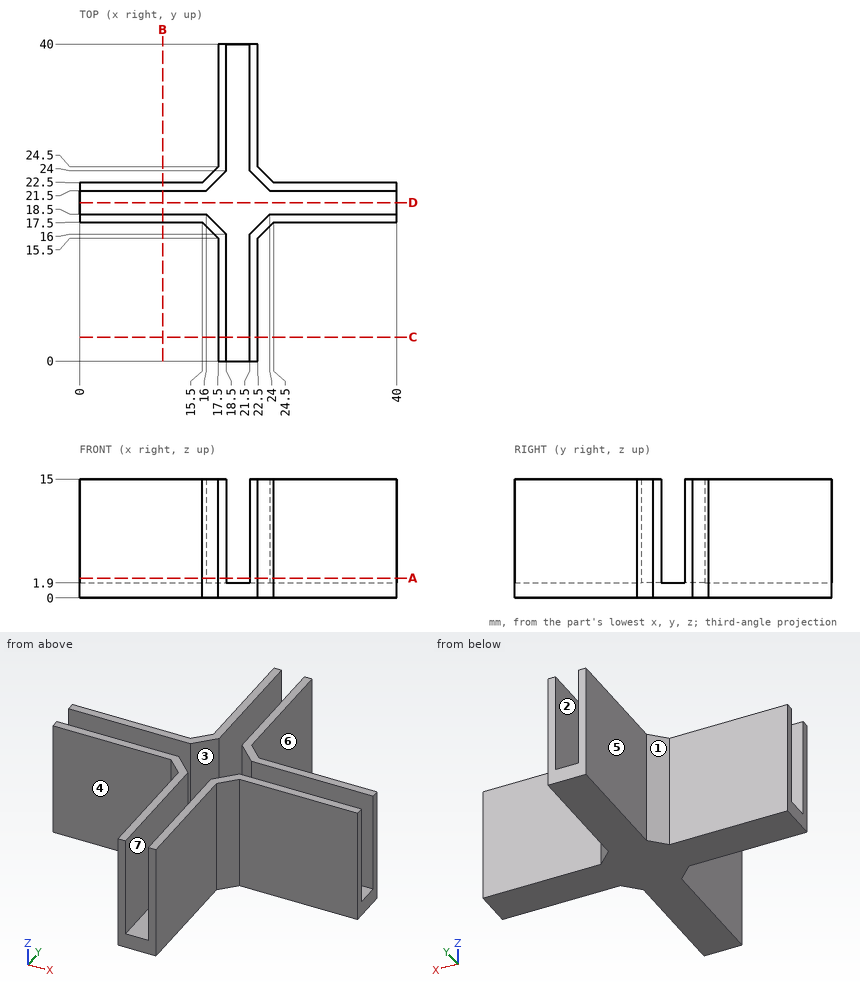
For this review, use the dimensioned drawing (mm, ordinates from the lowest corner) and the shaded views. A direction names the side the tool comes from. Coordinates: 2 decimals unless noted, no trailing zeros. Loops run counter-clockwise (first coordinate to the right, second up) from the corner with the lowest first, then second, coordinate; pieces in that order, holes last.
1. Add section A-A, the plane z = 2.5. Count the separate pieces of the cut face and the enclosed holes in it, then the cut area to 4 significant figures.
2. Add section D-D, the plane y = 20. Give the boundary of the cut face in (x, z), then the cut area to 3 significant figures.
3. For the marked faces 4, 5, 6 and 7, list the 3-axis set-ups (+Z, -Z, +X, -X, +Y, -Y) from which the entire face can be reached by the end or side of a thin tool; tool diameter is ignored.
4. Insertion check: P1, Ø6, axis at x = 14, z = 10.5, coming from the +Y side; P2, Ø6.5, axis at x = 8.5, z = 9.5, coming from the +Y side; P3, Ø7.5, axis at y = 4.5, z = 11, coming from the -X side; P4, Ø6, axis at y = 16.5, z = 2, coming from the +X side. Each pin has a flat end and moves straight along its axis. Give the tip position at first contact, or say it passes through.
5. Mouldability with a two-part tool opening along Y and no side actions: class the marked faces 1, 2 and 3 as +Y half, -Y half, draft (parallel to the pull), parting line (faces both ways), or undercut.
6. For line 1 (X direction, y = 35.5, z = 4.75); line 2 (X direction, y = 16.5, z = 7.75), list the stretches that pass through material, from the lowest coordinate up.
7. Add section B-B, the plane x = 10.5. Give the boundary of the cut face in (y, z).
Result:
1. separate pieces: 4
1. enclosed holes: 0
1. area: 139.5 mm2
2. outline: (0, 0) - (40, 0) - (40, 1.9) - (0, 1.9) - close
2. area: 76.0 mm2
3. face 4: +Z, -Z, -X, -Y
3. face 5: +Z, -Z, -X, +Y
3. face 6: +Z, -Z, +X, +Y
3. face 7: +Z, +Y, -Y
4. P1: stops at y = 24
4. P2: stops at y = 22.5
4. P3: stops at x = 17.5
4. P4: stops at x = 40
5. face 1: +Y half
5. face 2: draft
5. face 3: undercut
6. line 1: x = 17.5 to 18.5, 21.5 to 22.5
6. line 2: x = 16.5 to 18, 22 to 23.5
7. outline: (17.5, 0) - (22.5, 0) - (22.5, 15) - (21.5, 15) - (21.5, 1.9) - (18.5, 1.9) - (18.5, 15) - (17.5, 15) - close
